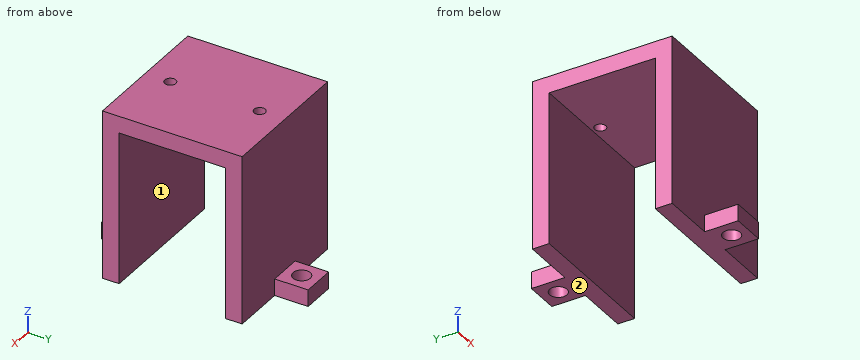
Autodesk Inventor part; units mm, degrees
ref_plane "YZ Plane" through (0, 0, 0) normal (1, 0, 0) x (0, 1, 0)
ref_plane "XZ Plane" through (0, 0, 0) normal (0, 1, 0) x (-1, 0, 0)
ref_plane "XY Plane" through (0, 0, 0) normal (0, 0, 1) x (1, 0, 0)
sketch "Sketch1" plane through (0, 0, 0) normal (0, 0, 1) x (1, 0, 0)
  line L0 (-12.5, 12.5) -> (12.5, 12.5)
  line L1 (12.5, 12.5) -> (12.5, -12.5)
  line L2 (12.5, -12.5) -> (-12.5, -12.5)
  line L3 (-12.5, -12.5) -> (-12.5, 12.5)
  line L4 (-12.5, 12.5) -> (12.5, -12.5) construction
  line L5 (12.5, 12.5) -> (-12.5, -12.5) construction
  point P0 (0, 0)
  dimension "d0" = 25
  dimension "d1" = 25
extrude "Extrusion1" add sketch "Sketch1" along normal blind 30.25
sketch "Sketch3" plane through (-12.5, -12.5, 0) normal (-1, 0, 0) x (0, 0, 1)
  line L0 (0, 25) -> (0, 0)
  line L1 (0, 25) -> (30.25, 25)
  line L2 (30.25, 0) -> (30.25, 25)
  line L3 (0, 0) -> (30.25, 0)
  line L4 (27.25, 3) -> (27.25, 22)
  line L5 (27.25, 22) -> (3, 22)
  line L6 (3, 3) -> (27.25, 3)
  line L7 (3, 3) -> (0, 3)
  line L8 (3, 22) -> (0, 22)
  line L9 (0, 3) -> (0, 22)
  line L10 (0, 0) -> (0, 25)
  point P0 (0, 12.5)
  dimension "d16" = 3
sketch "Sketch4" plane through (0, 0, 0) normal (0, 0, -1) x (-1, 0, 0)
  line L0 (3, 18.5) -> (-3, 18.5)
  line L1 (-3, 18.5) -> (-3, 12.5)
  line L2 (-3, 12.5) -> (3, 12.5)
  line L3 (3, 12.5) -> (3, 18.5)
  line L4 (3, 18.5) -> (-3, 12.5) construction
  line L5 (-3, 18.5) -> (3, 12.5) construction
  point P0 (0, 0)
  point P1 (0, 19)
  point P2 (0, 15.5)
  dimension "d19" = 6
  dimension "d20" = 6
extrude "Extrusion3" add sketch "Sketch4" against normal blind 3
mirror "Mirror1" about plane through (0, 0, 0) normal (0, 1, 0) of "Extrusion3"
extrude "Extrusion4" cut sketch "Sketch3" against normal up to next contours L8 L5 L4 L6 L7 L0
sketch "Sketch5" plane through (0, 0, 0) normal (0, 0, -1) x (-1, 0, 0)
  circle A0 centre (0, 15.5) radius 1.55
  point P0 (0, 0)
  dimension "d21" = 3.1
extrude "Extrusion5" cut sketch "Sketch5" against normal up to next
mirror "Mirror2" about plane through (0, 0, 0) normal (0, 1, 0) of "Extrusion5"
sketch "Sketch6" plane through (0, 0, 30.25) normal (0, 0, 1) x (1, 0, 0)
  circle A0 centre (0, -8) radius 1
  circle A1 centre (0, 8) radius 1
  point P0 (0, 0)
  dimension "d24" = 2
  dimension "d25" = 2
extrude "Extrusion6" cut sketch "Sketch6" against normal up to next
properties part number "架子 assembly"
Verification items for the finished model (mm, model axes). Face numbers are marked on the shaded views. A direction names the side the tool comes from. Round coordinates to 2 decimals unless told otherwise and drop trailing zeros. Loops run counter-clockwise (first coordinate to the right, second up) from the corner with the lowest first, then second, coordinate; pieces in that order, holes last. Notation, with made-up numbers: (48.5, 54) - (81.5, 54) arc R20 ccw to (81.5, 62) - close; hole circle Ø1 at (32.25, 36.5). An arc over 180 degrees is marked (long way). Use one line per item in the form item = value.
1. Gauge pin test, flat ends, axial feed: pin 1 Ø0.9 at (y, z) = (-14.5, 1) entering from +X; pin 2 Ø7.5 at (x, z) = (-4, 17.5) entering from +Y; pin 3 Ø2 at (x, z) = (4.5, 7) entering from -Y; pin 4 Ø1.2 at (x, y) = (0, 8) entering from +Z. Record the tip position at first contact, or that the pin passes through.
A:
pin_1 = 3
pin_2 = 12.5
pin_3 = -12.5
pin_4 = through
2. Section check C-C on z = 25. Record the cut outline in (x, y), and give its area (3 significant figures).
A:
outline = (-12.5, -12.5) - (12.5, -12.5) - (12.5, -9.5) - (-12.5, -9.5) - close; (-12.5, 9.5) - (12.5, 9.5) - (12.5, 12.5) - (-12.5, 12.5) - close
area = 150 mm²
3. Scan lines: probe 1 along Y at (x, z) = (0, 28.25); probe 2 along Y at (x, z) = (0, 1.65); probe 3 along Y at (x, z) = (-9.75, 22.5). Record each from-to range of solid material in increasing order.
A:
probe_1 = -12.5 to -9, -7 to 7, 9 to 12.5
probe_2 = -18.5 to -17.05, -13.95 to -9.5, 9.5 to 13.95, 17.05 to 18.5
probe_3 = -12.5 to -9.5, 9.5 to 12.5
4. Section check A-A on x = 0. Record the cut outline in (y, z).
A:
outline = (-18.5, 0) - (-17.05, 0) - (-17.05, 3) - (-18.5, 3) - close; (-13.95, 0) - (-9.5, 0) - (-9.5, 27.25) - (-9, 27.25) - (-9, 30.25) - (-12.5, 30.25) - (-12.5, 3) - (-13.95, 3) - close; (-7, 27.25) - (7, 27.25) - (7, 30.25) - (-7, 30.25) - close; (9, 27.25) - (9.5, 27.25) - (9.5, 0) - (13.95, 0) - (13.95, 3) - (12.5, 3) - (12.5, 30.25) - (9, 30.25) - close; (17.05, 0) - (18.5, 0) - (18.5, 3) - (17.05, 3) - close
5. Section check B-B on y = 8. Record the cut outline in (x, z).
A:
outline = (-12.5, 27.25) - (-1, 27.25) - (-1, 30.25) - (-12.5, 30.25) - close; (1, 27.25) - (12.5, 27.25) - (12.5, 30.25) - (1, 30.25) - close
6. Access from +Z, -Z, +X, -X, +Y, -Y to the whole of each face (thin tool, end or side, straight path). Record for the marked faces 1 and 2.
A:
face_1 = -Z, +X, -X
face_2 = -Z, +X, -X, +Y, -Y
7. Section check D-D on x = -2.5. Record the cut outline in (y, z).
A:
outline = (-18.5, 0) - (-9.5, 0) - (-9.5, 27.25) - (9.5, 27.25) - (9.5, 0) - (18.5, 0) - (18.5, 3) - (12.5, 3) - (12.5, 30.25) - (-12.5, 30.25) - (-12.5, 3) - (-18.5, 3) - close
